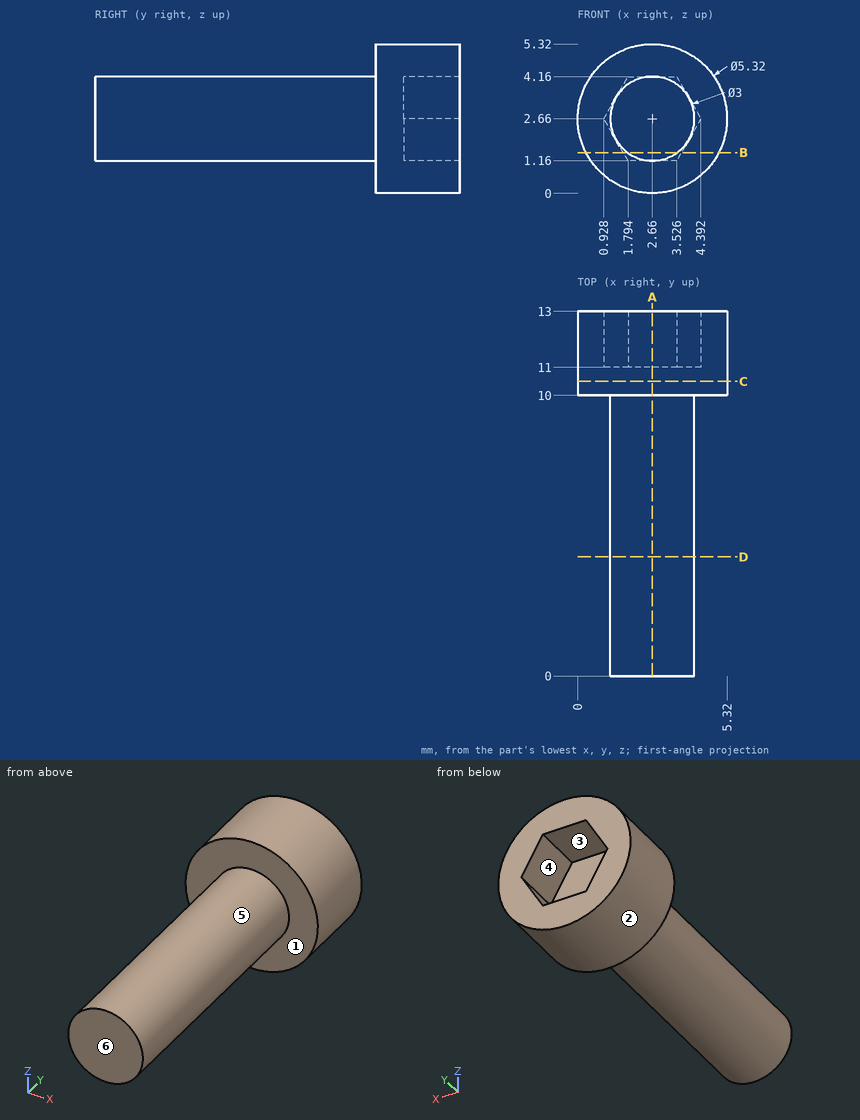
Check sheet for the drawn part. Datum: minimum x, y, z corner. Units: mm. A direction names the side the tool comes from. Round coordinates to 2 decimals unless told otherwise and drop trailing zeros. Loops run counter-clockwise (first coordinate to the right, second up) from the corner with the lowest first, then second, coordinate; pieces in that order, holes last. Notation, with made-up numbers: M 88.25,47 L 114.25,47 A24 cw 114.25,75 Z; hole C -27,43 d9. An arc over 180 degrees is marked long. Write each question's results on one line, items separated by ' | '.
1) Section check C-C on y = 10.5. Record the boundary of the cut face in (x, z).
Checks:
outline: C 2.66,2.66 d5.32
2) Section check B-B on z = 1.45. Record the boundary of the cut face in (x, y).
Checks:
outline: M 0.29,10 L 1.77,10 L 1.77,0 L 3.55,0 L 3.55,10 L 5.03,10 L 5.03,13 L 3.69,13 L 3.69,11 L 1.63,11 L 1.63,13 L 0.29,13 Z
3) Gauge pin test, flat ends, axial feed: P1, Ø2, axis at x = 2.5, y = 8, coming from the +Z side; P2, Ø1, axis at x = 2, y = 8.5, coming from the -Z side; P3, Ø2, axis at y = 9.5, z = 1, coming from the +X side. Record the tip position at first contact, or that the pin passes through.
Checks:
P1: stops at z = 4.16 | P2: stops at z = 1.17 | P3: stops at x = 5.2
4) Scan lines: L1, parallel to Z at x = 2.65, y = 6.5; L2, parallel to X at y = 11.25, z = 2.05; L3, parallel to Y at x = 0.6, z = 2.6. Record each from-to range of solid material in increasing order. Write a range as from..to.
Checks:
L1: z = 1.16..4.16 | L2: x = 0.07..1.28, 4.04..5.25 | L3: y = 10..13
5) Access from +Z, -Z, +X, -X, +Y, -Y to the whole of each face (thin tool, end or side, straight path). Record for the marked faces 4, 5 and 6.
Checks:
face 4: +Y | face 5: -Y | face 6: +Z, -Z, +X, -X, -Y
6) Section check D-D on y = 4.25. Record the boundary of the cut face in (x, z), then the cut area to 3 significant figures.
Checks:
outline: C 2.66,2.66 d3 | area: 7.07 mm2
7) Mould release check, pull along Z, two halves, no side actions. Record for the marked faces 1, 2 and 3: released by +Z, released by -Z, zero draft, split by the parting line, or undercut.
Checks:
face 1: zero draft | face 2: split by the parting line | face 3: undercut
8) Section check A-A on x = 2.66. Record the boundary of the cut face in (y, z).
Checks:
outline: M 0,1.16 L 10,1.16 L 10,0 L 13,0 L 13,1.16 L 11,1.16 L 11,4.16 L 13,4.16 L 13,5.32 L 10,5.32 L 10,4.16 L 0,4.16 Z
